Part print with two shaded views. Sizes in mm from the minimum x, y, z corner. Coordinates: 2 decimals unless noted, no trailing zeros. Write each loop counter-clockwise with the first axis right and the second up, starting at its lowest first coordinate (ties: lowest second). Pieces come first, ordered by that corner, then holes.
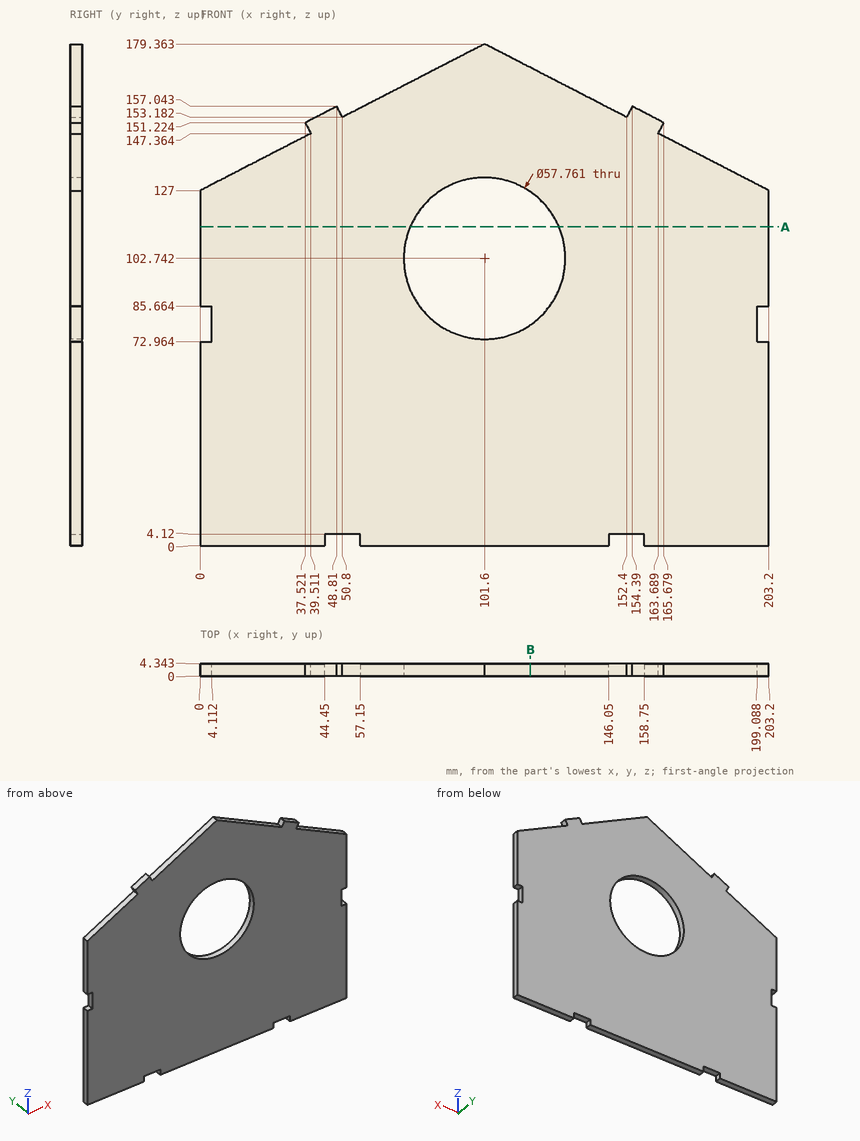
(1) Slice it at A-A, the plane z = 114. List the corners of the cut face in (x, y).
(2) Slice it at B-B, the plane x = 118. List the corners of the cut face in (y, z) (1 decimal).
(3) Probe L1, parallel to Z at x = 101.6, y = 0.95 (1 decimal); L2, parallel to Z at x = 103.5, y = 1.3 (1 decimal); L3, parallel to X at y = 2.05, z = 104.5. List the from-to ranges inside material, lowest first.
(4) Flat gauge pins, fed straight in: P1, Ø1.3, axis at y = 2.5, z = 81, coming from the -X side; P2, Ø1, axis at y = 1.5, z = 79.5, coming from the +X side; P3, Ø1.5, axis at x = 104, y = 3, coming from the +Z side. Where does each tip first touch, or does it go through?
Results:
1. outline: (0, 0) - (75, 0) - (75, 4.34) - (0, 4.34) - close; (128.2, 0) - (203.2, 0) - (203.2, 4.34) - (128.2, 4.34) - close
2. outline: (0, 0) - (4.3, 0) - (4.3, 79) - (0, 79) - close; (0, 126.5) - (4.3, 126.5) - (4.3, 170.9) - (0, 170.9) - close
3. L1: z = 0 to 73.9, 131.6 to 179.4
3. L2: z = 0 to 73.9, 131.6 to 178.4
3. L3: x = 0 to 72.77, 130.43 to 203.2
4. P1: stops at x = 4.11
4. P2: stops at x = 199.09
4. P3: stops at z = 178.51
